Could you check a few things on this model? Use its own coordinates, in mm. Coordinates: 2 decimals unless noted, no trailing zeros. Write each loop counter-clockwise with the first axis right and the second up, starting at its lowest first coordinate (ties: lowest second). Pieces come first, ordered by that corner, then holes.
```python
from build123d import *

# Parameters (mm, degrees)
BOX_W               = 80
BOX_H               = 10
BOX_DEPTH           = 10
BOX_ROLL_ANGLE      = 78.842738
BOX_PITCH_ANGLE     = 38.475947
BOX_PLACEMENT_ANGLE = 38.177648


with BuildPart() as part:
    # Box → Box (new body)
    with BuildSketch(Plane.XY):
        with Locations((40, 5)):
            Rectangle(BOX_W, BOX_H)
    extrude(amount=BOX_DEPTH)


with BuildPart() as part_1:
    # Box roll: moved
    add(part.part.rotate(Axis((0, 0, 0), (1, 0, 0)), BOX_ROLL_ANGLE))


with BuildPart() as part_2:
    # Box pitch: moved
    add(part_1.part.rotate(Axis((0, 0, 0), (0, 1, 0)), BOX_PITCH_ANGLE))


with BuildPart() as part_3:
    # Box placement: moved
    add(part_2.part.rotate(Axis((0, 0, 0), (0, 0, 1)), BOX_PLACEMENT_ANGLE))


solid = part_3.part
```
1. For pin 1 (2 mm diameter, centred on x = 47.5, y = 34.5, fed in from +Z); pin 2 (3 mm diameter, centred on y = 18.5, z = -23, fed in from -X); pin 3 (3 mm diameter, centred on y = 20.5, z = -25.5, fed in from -X), each with a flat end and sliding along its axis, tell me the tip position at first contact or that it passes through.
Verdict:
pin 1: stops at z = -32.21
pin 2: stops at x = 21.93
pin 3: stops at x = 24.45
2. I want a section at B-B on x = 37.5. Please give me the cut outline in (y, z), plus the area to 3 significant figures.
Verdict:
outline: (17.01, -29.31) - (29.49, -37.91) - (31.95, -26.59) - (19.47, -17.99) - close
area: 162 mm2
3. Please list where these lines run through material, in increasing order: line 1 along Y through (x, z) = (40, -40); line 2 along Z through (x, y) = (54, 34); line 3 along Z through (x, y) = (22.5, 14.5).
Verdict:
line 1: y = 30.81 to 31.55
line 2: z = -48.72 to -35.74
line 3: z = -20.55 to -7.53
4. I want a section at A-A on z = -30. Please give me the cut outline in (x, y), plus the area to 3 significant figures.
Verdict:
outline: (29.67, 23.33) - (38.18, 17.54) - (49.38, 28.81) - (40.87, 34.6) - close
area: 161 mm2
